Autodesk Inventor part; units mm, degrees
ref_plane "YZ Plane" through (0, 0, 0) normal (1, 0, 0) x (0, 1, 0)
ref_plane "XZ Plane" through (0, 0, 0) normal (0, 1, 0) x (-1, 0, 0)
ref_plane "XY Plane" through (0, 0, 0) normal (0, 0, 1) x (1, 0, 0)
sketch "Sketch1" plane through (0, 0, 0) normal (0, 0, 1) x (1, 0, 0)
  line L0 (0, 0) -> (10, 0)
  line L1 (10, 0) -> (10, -27.5)
  line L2 (10, -27.5) -> (23.0834, -27.5)
  line L3 (23.0834, -27.5) -> (28.1466, 0)
  line L4 (28.1466, 0) -> (39.1466, 0)
  line L5 (39.1466, 0) -> (46.1888, -34.158)
  line L6 (38.0632, -45.4132) -> (38.0632, -35)
  line L7 (38.0632, -35) -> (0, -35)
  line L8 (0, -35) -> (0, 0)
  line L9 (46.1888, -34.158) -> (46.1888, -45.4132)
  line L10 (46.1888, -45.4132) -> (38.0632, -45.4132)
  line L11 (28.1466, 0) -> (33.3359, 28.1848) construction
  line L12 (33.3359, 28.1848) -> (39.1466, 0) construction
  line L13 (28.1466, 0) -> (28.5149, 2)
  line L14 (38.7343, 2) -> (39.1466, 0)
  line L15 (38.7343, 2) -> (28.5149, 2)
  point P0 (4.5, -10)
  point P1 (4.5, -25)
  point P2 (42.126, -41.9632)
  point P3 (33.6466, -1.9132)
  point P4 (38.0632, -40.2066)
  point P5 (42.126, -45.4132)
  point P6 (33.6466, 0)
  dimension "d0" = 35
  dimension "d1" = 10
  dimension "d2" = 10
  dimension "d3" = 4.5
  dimension "d4" = 100.432
  dimension "d6" = 101.649
  dimension "d7" = 7.5
  dimension "d8" = 15
  dimension "d9" = 8.1256
  dimension "d10" = 38.0632
  dimension "d11" = 10.4132
  dimension "d12" = 3.45
  dimension "d13" = 1.9132
  dimension "d14" = 29.1466
  dimension "d15" = 28.1848
  dimension "d30" = 2
extrude "Extrusion1" add sketch "Sketch1" along normal blind 5
hole "Hole1" at (4.5, -10, 0) at (4.5, -25, 0) at (42.126, -41.9632, 0) at (33.6466, -1.9132, 0) direction (0, 0, 1) diameter 3 depth 20
sketch "Sketch2" plane through (0, 0, 5) normal (0, 0, 1) x (1, 0, 0)
  circle A0 centre (33.6466, -1.9132) radius 1.5
  circle A1 centre (42.126, -41.9632) radius 1.5
  circle A2 centre (4.5, -25) radius 1.5
  circle A3 centre (4.5, -10) radius 1.5
  line L0 (0, -35) -> (38.0632, -35)
  line L1 (38.0632, -35) -> (38.0632, -45.4132)
  line L2 (38.0632, -45.4132) -> (46.1888, -45.4132)
  line L3 (46.1888, -45.4132) -> (46.1888, -34.158)
  line L4 (23.0834, -27.5) -> (10, -27.5)
  line L5 (10, -27.5) -> (10, 0)
  line L6 (10, 0) -> (0, 0)
  line L7 (0, 0) -> (0, -35)
  line L8 (35.2921, 0.9368) -> (36.9375, -1.9132)
  line L9 (36.9375, -1.9132) -> (35.2921, -4.7632)
  line L10 (35.2921, -4.7632) -> (32.0012, -4.7632)
  line L11 (32.0012, -4.7632) -> (30.3557, -1.9132)
  line L12 (30.3557, -1.9132) -> (32.0012, 0.9368)
  line L13 (32.0012, 0.9368) -> (35.2921, 0.9368)
  line L14 (43.7715, -39.1132) -> (45.4169, -41.9632)
  line L15 (45.4169, -41.9632) -> (43.7715, -44.8132)
  line L16 (43.7715, -44.8132) -> (40.4806, -44.8132)
  line L17 (40.4806, -44.8132) -> (38.8351, -41.9632)
  line L18 (38.8351, -41.9632) -> (40.4806, -39.1132)
  line L19 (40.4806, -39.1132) -> (43.7715, -39.1132)
  line L20 (46.1888, -34.158) -> (38.7343, 2)
  line L21 (38.7343, 2) -> (28.5149, 2)
  line L22 (28.5149, 2) -> (23.0834, -27.5)
  dimension "d25" = 6.5818
  dimension "d26" = 6.5818
extrude "Extrusion2" cut sketch "Sketch2" against normal blind 4 contours L8 L9 L10 L11 L12 L13 | L14 L15 L16 L17 L18 L19
fillet "Fillet1" radius 2 11 edges at (0, 0, 2.5) (10, 0, 2.5) (10, -27.5, 2.5) (23.0834, -27.5, 2.5) (0, -35, 2.5) (38.0632, -35, 2.5) (38.0632, -45.4132, 2.5) (46.1888, -45.4132, 2.5) (46.1888, -34.158, 2.5) (28.5149, 2, 2.5) (38.7343, 2, 2.5)
properties part number "FanMountV2" material "ABS Plastic"
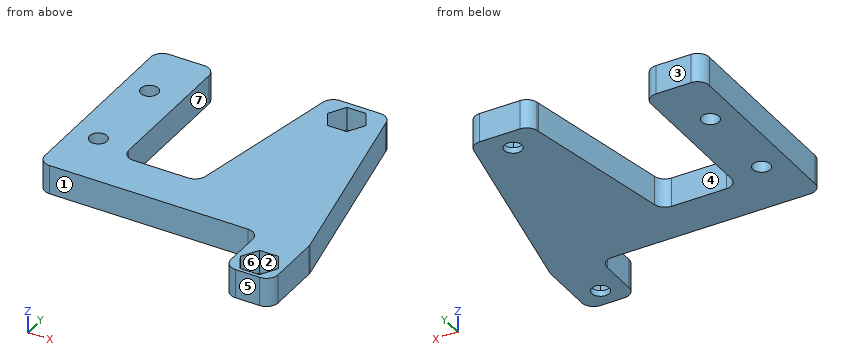
Verification items for the finished model (mm, model axes). Face numbers are marked on the shaded views. A direction names the side the tool comes from. Coordinates: 2 decimals unless noted, no trailing zeros. Order: outer loops, then holes, each group sorted by start corner. A loop starts at its lowest first (then second) coordinate and runs counter-clockwise, first axis right, second up. Notation, with made-up numbers: (-18.5, 43.5) -> (40.5, 43.5) arc R20 ccw to (40.5, 53.5) -> close; hole circle Ø3 at (17.5, 48). An arc over 180 degrees is marked (long way). Answer as CSV lines item,"result". Start each with the question number.
1) Gauge pin test, flat ends, axial feed: pin 1 Ø1.5 at (y, z) = (-22.5, 4.5) entering from +X; pin 2 Ø2.5 at (x, y) = (4.5, -25) entering from -Z; pin 3 Ø1.5 at (x, z) = (16.5, 3.5) entering from -Y; pin 4 Ø1.5 at (x, z) = (5, 3.5) entering from +Y. Record the tip position at first contact, or that the pin passes through.
2) Release check for a two-part mould opening along Y. For the marked faces 5, 6 and 7 record: released by +Y, released by -Y, zero draft, split by the parting line, or undercut.
3) Material ranges on L1, parallel to Y at x = 4.5, z = 3.95; L2, parallel to X at y = -9, z = 4.4; L3, parallel to X at y = -25, z = 2.1, recorded low to high. Write a range as [from, to].
4) Cross-section at A-A, the plane y = -13. Record the boundary of the cut face in (x, z), then the cut area to 3 significant figures.
5) Cross-section at B-B, the plane x = 4.5. Record the boundary of the cut face in (y, z), then the cut area to 3 significant figures.
6) Cross-section at D-D, the plane z = 4.25. Give the number of separate pieces and of enclosed holes in the cut face, then the cut area to 3 significant figures.
7) Set-up check for the marked faces 1, 2, 3 and 4: record each of +Z, -Z, +X, -X, +Y, -Y from which the full face is reachable in a straight line by a thin tool's end or side.
8) Cross-section at C-C, the plane x = 33. Record the boundary of the cut face in (y, z).
Conclusion:
1,pin 1,"stops at x = 43.94"
1,pin 2,"passes through"
1,pin 3,"stops at y = -35"
1,pin 4,"stops at y = 0"
2,face 5,"released by -Y"
2,face 6,"undercut"
2,face 7,"zero draft"
3,L1,"y = [-35, -26.5], [-23.5, -11.5], [-8.5, 0]"
3,L2,"x = [0, 3.38], [5.62, 10], [26.49, 41]"
3,L3,"x = [0, 3], [6, 10], [23.54, 44.3]"
4,outline,"(0, 0) -> (10, 0) -> (10, 5) -> (0, 5) -> close; (25.75, 0) -> (41.83, 0) -> (41.83, 5) -> (25.75, 5) -> close"
4,area,"130 mm²"
5,outline,"(-35, 0) -> (-26.5, 0) -> (-26.5, 5) -> (-35, 5) -> close; (-23.5, 0) -> (-11.5, 0) -> (-11.5, 5) -> (-23.5, 5) -> close; (-8.5, 0) -> (0, 0) -> (0, 5) -> (-8.5, 5) -> close"
5,area,"145 mm²"
6,separate pieces,"1"
6,enclosed holes,"4"
6,area,"1,100 mm²"
7,face 1,"+Z, -Z, -X, -Y"
7,face 2,"+Z"
7,face 3,"+Z, -Z, -X, +Y"
7,face 4,"+Z, -Z, +Y"
8,outline,"(-35, 0) -> (-3.27, 0) -> (-3.27, 1) -> (-4.76, 1) -> (-4.76, 5) -> (-35, 5) -> close; (-0.56, 0) -> (2, 0) -> (2, 5) -> (0.94, 5) -> (0.94, 1) -> (-0.56, 1) -> close"
